```python
from build123d import *

# Parameters (mm, degrees)
ESBO_O1_W                = 30
ESBO_O1_H                = 50
ESBO_O1_W_2              = 28
ESBO_O1_H_2              = 48
EXTRUS_O_FINA1_DEPTH     = 60
RESSALTO_EXTRUS_O1_DEPTH = 60
ESBO_O3_R                = 1.5
CORTE_EXTRUS_O1_DEPTH    = 10


with BuildPart() as part:
    # Esboço1 → Extrusão-Fina1 (new body)
    with BuildSketch(Plane.XY):
        with Locations((-15, 25)):
            Rectangle(ESBO_O1_W, ESBO_O1_H)
        with Locations((-15, 25)):
            Rectangle(ESBO_O1_W_2, ESBO_O1_H_2, mode=Mode.SUBTRACT)
    extrude(amount=EXTRUS_O_FINA1_DEPTH)

    # Esboço2 → Ressalto-extrusão1 (add, through all)
    with BuildSketch(Plane(origin=(0, 0, 0), x_dir=(-1, 0, 0), z_dir=(0, 0, -1))):
        Polygon((0, 50), (1.071296322, 56.157995634), (2.075314272, 55.983328291), (1.034404539, 50), align=None)
    extrude(amount=-RESSALTO_EXTRUS_O1_DEPTH)

    # Esboço3 → Corte-extrusão1 (cut)
    with BuildSketch(Plane(origin=(0, 0, 0), x_dir=(0, 0, -1), z_dir=(1, 0, 0))):
        with Locations((-55, 35)):
            Circle(ESBO_O3_R)
        with Locations((-5, 35)):
            Circle(ESBO_O3_R)
    extrude(amount=-CORTE_EXTRUS_O1_DEPTH, mode=Mode.SUBTRACT)


solid = part.part
```
For this review, take the finished solid that the model builds, in its own axes (mm). A direction names the side the tool comes from. Give positions to 0.01 mm unless a question says otherwise; leave off trailing zeros. Order: outer loops, then holes, each group sorted by start corner. A loop starts at its lowest first (then second) coordinate and runs counter-clockwise, first axis right, second up.
1) Take a section at C-C (z = 22.5). Give the boundary of the cut face in (x, y), then the cut area to 3 significant figures.
2) The part is to be moulded in two halves that separate along Y. For faces 4 (the face through (-0.6, 34.4, 0)), 5 (the face through (-1.56, 53.03, 29.58)), 6 (the face through (-0.53, 53.04, 29.58)), say which applies: released by +Y, released by -Y, zero draft, split by the parting line, or undercut.
3) Take a section at B-B (y = 16). Give the boundary of the cut face in (x, z), then the cut area to 3 significant figures.
4) Take a section at A-A (x = -3.5). Give the boundary of the cut face in (y, z).
5) For faces 1 (the face through (-1, 25, 30)), 2 (the face through (0, 25, 30)), 3 (the face through (-0.493, 33.536, 5.325)), list the 3-axis set-ups (+Z, -Z, +X, -X, +Y, -Y) from which the entire face can be reached by the end or side of a thin tool; tool diameter is ignored.
6) Take a section at D-D (y = 35). Give the boundary of the cut face in (x, z).
7) Wall thickness on line 1 (Y direction, x = -4, z = 50.5); line 2 (X direction, y = 40.5, z = 32.5); line 3 (X direction, y = 53, z = 54.5): over which ranges is each line inside the solid? List them lowest first.
8) Insertion check: pin 1 (3 mm diameter, centred on x = -10.5, z = 25, fed in from +Y). The pin has a flat end and moves straight along its axis. Give the tip position at first contact, or say it passes through.
Derived:
1. outline: (-30, 0) - (0, 0) - (0, 50) - (-1.07, 56.16) - (-2.08, 55.98) - (-1.03, 50) - (-30, 50) - close; hole (-29, 1) - (-1, 1) - (-1, 49) - (-29, 49) - close
1. area: 162 mm2
2. face 4: zero draft
2. face 5: undercut
2. face 6: released by +Y
3. outline: (-30, 0) - (-29, 0) - (-29, 60) - (-30, 60) - close; (-1, 0) - (0, 0) - (0, 60) - (-1, 60) - close
3. area: 120 mm2
4. outline: (0, 0) - (1, 0) - (1, 60) - (0, 60) - close; (49, 0) - (50, 0) - (50, 60) - (49, 60) - close
5. face 1: +Z, -Z
5. face 2: +Z, -Z, +X, +Y, -Y
5. face 3: +X
6. outline: (-30, 0) - (-29, 0) - (-29, 60) - (-30, 60) - close; (-1, 0) - (0, 0) - (0, 3.5) - (-1, 3.5) - close; (-1, 6.5) - (0, 6.5) - (0, 53.5) - (-1, 53.5) - close; (-1, 56.5) - (0, 56.5) - (0, 60) - (-1, 60) - close
7. line 1: y = 0 to 1, 49 to 50
7. line 2: x = -30 to -29, -1 to 0
7. line 3: x = -1.56 to -0.52
8. pin 1: stops at y = 50
